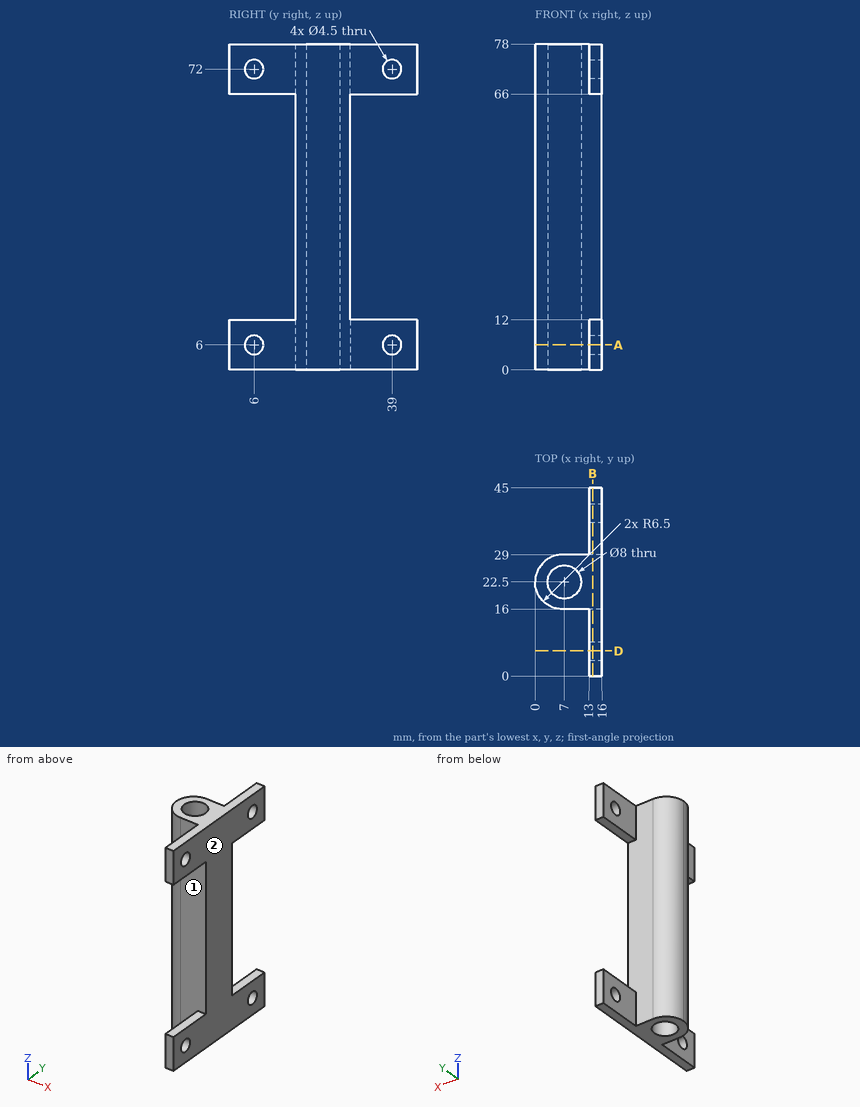
Here's the drawing with two shaded views (mm, measured from the low corner). I have some questions. Give positions to 0.01 mm unless a question says otherwise; leave off trailing zeros. Order: outer loops, then holes, each group sorted by start corner. A loop starts at its lowest first (then second) coordinate and runs counter-clockwise, first axis right, second up. Notation, with made-up numbers: (74, 32) -> (124, 32) arc R25 cw to (124, 70) -> close; hole circle Ø8 at (-23, 71). An arc over 180 degrees is marked (long way). Use a Markdown table: item, result. Add a question column.
Item 1: I need wall thicknesses on line 1 (Z direction, x = 14.55, y = 39); line 2 (Y direction, x = 14.5, z = 72); line 3 (Z direction, x = 15.75, y = 14.5). Which ranges of each line are inside material? Lowest first, please.
Item 2: Imagine slicing it at D-D on y = 6. Please give me the cut outline in (x, z).
Item 3: If we mould it in two halves opening along Z, with no side actions, what happens to the marked faces 1 and 2? For each: pulls with the +Z half, pulls with the -Z half, needs draft (parallel to the pull), parting line crosses it, or undercut.
Item 4: Will these pins go through, and if not, where does the flat tip stop? pin 1 (2 mm diameter, centred on x = 4.5, y = 24, fed in from +Z); pin 2 (8 mm diameter, centred on x = 11.5, y = 40, fed in from -Z); pin 3 (13 mm diameter, centred on y = 11, z = 4.5, fed in from -X); pin 4 (3.5 mm diameter, centred on y = 9.5, z = 71.5, fed in from -X).
Item 5: Imagine slicing it at A-A on z = 6. Give the number of separate pieces and of enclosed holes in the cut face, plus the area to 3 significant figures.
Item 6: Imagine slicing it at B-B on x = 13.75. Please give me the cut outline in (y, z).
Data:
| question | item | result |
|---|---|---|
| 1 | line 1 | z = 0 to 3.75, 8.25 to 12, 66 to 69.75, 74.25 to 78 |
| 1 | line 2 | y = 0 to 3.75, 8.25 to 36.75, 41.25 to 45 |
| 1 | line 3 | z = 0 to 12, 66 to 78 |
| 2 | outline | (13, 0) -> (16, 0) -> (16, 3.75) -> (13, 3.75) -> close; (13, 8.25) -> (16, 8.25) -> (16, 12) -> (13, 12) -> close; (13, 66) -> (16, 66) -> (16, 69.75) -> (13, 69.75) -> close; (13, 74.25) -> (16, 74.25) -> (16, 78) -> (13, 78) -> close |
| 3 | face 1 | undercut |
| 3 | face 2 | needs draft |
| 4 | pin 1 | passes through |
| 4 | pin 2 | stops at z = 0 |
| 4 | pin 3 | stops at x = 2.35 |
| 4 | pin 4 | stops at x = 13 |
| 5 | separate pieces | 3 |
| 5 | enclosed holes | 1 |
| 5 | area | 209 mm² |
| 6 | outline | (0, 0) -> (45, 0) -> (45, 12) -> (29, 12) -> (29, 66) -> (45, 66) -> (45, 78) -> (0, 78) -> (0, 66) -> (16, 66) -> (16, 12) -> (0, 12) -> close; hole circle Ø4.5 at (6, 6); hole circle Ø4.5 at (6, 72); hole circle Ø4.5 at (39, 6); hole circle Ø4.5 at (39, 72) |
